Input: part model. Units: mm. Frame: model coordinates. A direction names the side the tool comes from. Coordinates: 2 decimals unless noted, no trailing zeros. Loops run counter-clockwise (first coordinate to the right, second up) from the corner with the lowest first, then second, coordinate; pieces in that order, holes last. Notation, with made-up numbers: (86.5, 31.5) -> (96.5, 31.5) arc R25 ccw to (96.5, 63.5) -> close; hole circle Ø7 at (13.25, 55). An arc over 180 degrees is marked (long way). Answer as a JSON object with one key per item and string values.
from build123d import *

# Parameters (mm, degrees)
F1_DEPTH = 12.7
F2_R     = 3.96875
F3_DEPTH = 12.701
F4_R     = 9.525
F5_R     = 1.5875


with BuildPart() as f1:
    # F0 (on Top) → F1 (new body)
    with BuildSketch(Plane.XY):
        with BuildLine():
            Line((-19.247415, 16.8275), (-9.715362, 16.8275))
            Line((-9.715362, 16.8275), (9.715362, 16.8275))
            Line((9.715362, 16.8275), (19.430723, 0))
            Line((19.430723, 0), (9.715362, -16.8275))
            Line((9.715362, -16.8275), (-9.715362, -16.8275))
            Line((-9.715362, -16.8275), (-18.879693, -16.8275))
            ThreePointArc((-18.879693, -16.8275), (8.495577, -31.687447), (33.187688, -12.7))
            Line((33.187688, -12.7), (101.6, -12.7))
            ThreePointArc((101.6, -12.7), (88.9, 0), (101.6, 12.7))
            Line((101.6, 12.7), (33.63367, 12.7))
            ThreePointArc((33.63367, 12.7), (8.588902, 32.646256), (-19.247415, 16.8275))
        make_face()
        with BuildLine():
            ThreePointArc((114.3, 0), (110.580256, 8.980256), (101.6, 12.7))
            ThreePointArc((101.6, 12.7), (88.9, 0), (101.6, -12.7))
            ThreePointArc((101.6, -12.7), (110.580256, -8.980256), (114.3, 0))
        make_face()
    extrude(amount=F1_DEPTH)

    # F2 (on face) → F3 (cut, through all)
    with BuildSketch(Plane.XY.offset(12.7)):
        with Locations((101.6, 0)):
            Circle(F2_R)
    extrude(amount=-F3_DEPTH, mode=Mode.SUBTRACT)

    # F4
    f4_edges = [f1.edges().sort_by_distance(p)[0] for p in [
        (33.63367, 12.7, 6.35),
        (33.187688, -12.7, 6.35),
    ]]
    fillet(f4_edges, radius=F4_R)

    # F5
    f5_edges = [f1.edges().sort_by_distance(p)[0] for p in [
        (-19.247415, 16.8275, 6.35),
        (-18.879693, -16.8275, 6.35),
    ]]
    fillet(f5_edges, radius=F5_R)


solid = f1.part
1. Pin query (flat end, axial travel): P1, Ø1, axis at y = -25, z = 8, coming from the -X side; P2, Ø6.5, axis at x = -7.5, z = 8, coming from the +Y side; P3, Ø6.5, axis at x = 75, z = 5.5, coming from the +Y side; P4, Ø7, axis at x = 101.6, y = 0, coming from the -Z side. Return the tip coordinate at first contact, or that it passes through.
Reply:
{"P1": "stops at x = -12.81", "P2": "stops at y = 30.69", "P3": "stops at y = 12.7", "P4": "passes through"}
2. Section query C-C (x = 71). Return loops of the section in (y, z).
Reply:
{"outline": "(-12.7, 0) -> (12.7, 0) -> (12.7, 12.7) -> (-12.7, 12.7) -> close"}
3. Section query B-B (x = 12). Return loops of the section in (y, z), plus the area to 3 significant figures.
Reply:
{"outline": "(-31.19, 0) -> (-12.87, 0) -> (-12.87, 12.7) -> (-31.19, 12.7) -> close; (12.87, 0) -> (32.17, 0) -> (32.17, 12.7) -> (12.87, 12.7) -> close", "area": "478 mm2"}
4. Mould query, pull axis Y, two halves, no side actions, for faces 1 (the face through (71, 12.7, 6)), 2 (the face through (14.505, 8.532, 6.261)), 3 (the face through (47, 1, 12.7)), 4 (the face through (-3, -16.828, 6)). Classes: pulls with the +Y half, pulls with the -Y half, needs draft (parallel to the pull), parting line crosses it, or undercut.
Reply:
{"face 1": "pulls with the +Y half", "face 2": "undercut", "face 3": "needs draft", "face 4": "undercut"}
5. Section query D-D (y = 8). Return loops of the section in (x, z).
Reply:
{"outline": "(14.81, 0) -> (111.46, 0) -> (111.46, 12.7) -> (14.81, 12.7) -> close"}
6. Access query for faces 5 (the face through (14.64, -8.3, 6.26)), 6 (the face through (70, -12.7, 6)), 7 (the face through (97.635, 0.174, 6.439)). Directions: +Z, -Z, +X, -X, +Y, -Y. A direction counts if a zero-diameter tool reaches every point of the face in a straight line with its end or side. Return the directions, or none.
Reply:
{"face 5": "+Z, -Z, -X", "face 6": "+Z, -Z, +X, -Y", "face 7": "+Z, -Z"}
7. Line query: line 1 along Y through (x, z) = (101.6, 8.75); line 2 along Y through (x, z) = (46.5, 11); line 3 along X through (y, z) = (-0.5, 4). Output: solid intervals per line, ascending.
Reply:
{"line 1": "y = -12.7 to -3.97, 3.97 to 12.7", "line 2": "y = -12.7 to 12.7", "line 3": "x = 19.14 to 97.66, 105.54 to 114.29"}
